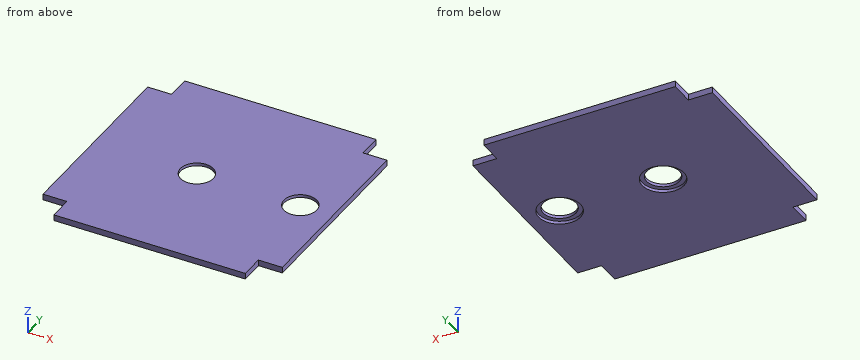
```python
from build123d import *

# Parameters (mm, degrees)
SKETCH1_W           = 100
SKETCH1_H           = 100
BOSS_EXTRUDE1_DEPTH = 2.5
SKETCH4_R           = 6.875
CUT_EXTRUDE2_DEPTH  = 142.443451598
SKETCH5_R           = 8.75
CUT_EXTRUDE3_DEPTH  = 1.25
SKETCH6_W           = 10
SKETCH6_H           = 10
CUT_EXTRUDE4_DEPTH  = 142.443451598


with BuildPart() as part:
    # Sketch1 → Boss-Extrude1 (new body)
    with BuildSketch(Plane.XY):
        with Locations((50, 50)):
            Rectangle(SKETCH1_W, SKETCH1_H)
    extrude(amount=BOSS_EXTRUDE1_DEPTH)

    # Sketch4 → Cut-Extrude2 (cut, through all)
    with BuildSketch(Plane.XY.offset(2.5)):
        with Locations((86.250042234, 48.943031999)):
            Circle(SKETCH4_R)
        with Locations((43.000042234, 48.943031999)):
            Circle(SKETCH4_R)
    extrude(amount=-CUT_EXTRUDE2_DEPTH, mode=Mode.SUBTRACT)

    # Sketch5 → Cut-Extrude3 (cut)
    with BuildSketch(Plane(origin=(0, 0, 0), x_dir=(-1, 0, 0), z_dir=(0, 0, -1))):
        with Locations((-86.250042234, 48.943031999)):
            Circle(SKETCH5_R)
        with Locations((-43.000042234, 48.943031999)):
            Circle(SKETCH5_R)
    extrude(amount=-CUT_EXTRUDE3_DEPTH, mode=Mode.SUBTRACT)

    # Sketch6 → Cut-Extrude4 (cut, through all)
    with BuildSketch(Plane(origin=(0, 0, 0), x_dir=(-1, 0, 0), z_dir=(0, 0, -1))):
        with Locations((-95, 95)):
            Rectangle(SKETCH6_W, SKETCH6_H)
        with Locations((-95, 5)):
            Rectangle(SKETCH6_W, SKETCH6_H)
        with Locations((-5, 95)):
            Rectangle(SKETCH6_W, SKETCH6_H)
        with Locations((-5, 5)):
            Rectangle(SKETCH6_W, SKETCH6_H)
    extrude(amount=-CUT_EXTRUDE4_DEPTH, mode=Mode.SUBTRACT)


solid = part.part
```
Can you work these out from the model? Positions are in its coordinate system, mm. Give positions to 0.01 mm unless a question says otherwise; leave off trailing zeros. Write each loop counter-clockwise with the first axis right and the second up, starting at its lowest first coordinate (ties: lowest second). Pieces come first, ordered by that corner, then holes. Notation, with made-up numbers: (-4.75, -34.75) - (51.25, -34.75) arc R22 ccw to (51.25, -9.75) - close; hole circle Ø7 at (-25.5, 12.25). An arc over 180 degrees is marked (long way). Write item = value, one per line. Start each with the question number.
1. Imagine slicing it at D-D (x = 84.5). Please give me the cut outline in (y, z).
2. Please list where these lines run through material, in increasing order: line 1 (X direction, y = 53.5, z = 1.65); line 2 (X direction, y = 46, z = 1.15); line 3 (Y direction, x = 8, z = 2.4).
3. Imagine slicing it at C-C (x = 8). Please give me the cut outline in (y, z).
4. Imagine slicing it at A-A (z = 1.8). Please give me the cut outline in (x, y) (3 decimals).
5. Imagine slicing it at B-B (x = 43.5). Please give me the cut outline in (y, z).
6. For pin 1 (0.8 mm diameter, centred on y = 5.5, z = 1, fed in from -X); pin 2 (1.2 mm diameter, centred on x = 7.5, z = 1.5, fed in from +Y); pin 3 (1.2 mm diameter, centred on x = 5, z = 1, fed in from -Y), each with a flat end and sliding along its axis, tell me the tip position at first contact or that it passes through.
Worked answers:
q1.outline = (0, 0) - (40.37, 0) - (40.37, 1.25) - (42.29, 1.25) - (42.29, 2.5) - (0, 2.5) - close; (55.59, 1.25) - (57.52, 1.25) - (57.52, 0) - (100, 0) - (100, 2.5) - (55.59, 2.5) - close
q2.line_1 = 0 to 37.85, 48.15 to 81.1, 91.4 to 100
q2.line_2 = 0 to 34.76, 51.24 to 78.01, 94.49 to 100
q2.line_3 = 10 to 90
q3.outline = (10, 0) - (90, 0) - (90, 2.5) - (10, 2.5) - close
q4.outline = (0, 10) - (10, 10) - (10, 0) - (90, 0) - (90, 10) - (100, 10) - (100, 90) - (90, 90) - (90, 100) - (10, 100) - (10, 90) - (0, 90) - close; hole circle Ø13.75 at (43, 48.943); hole circle Ø13.75 at (86.25, 48.943)
q5.outline = (0, 0) - (40.21, 0) - (40.21, 1.25) - (42.09, 1.25) - (42.09, 2.5) - (0, 2.5) - close; (55.8, 1.25) - (57.68, 1.25) - (57.68, 0) - (100, 0) - (100, 2.5) - (55.8, 2.5) - close
q6.pin_1 = 10
q6.pin_2 = 90
q6.pin_3 = 10
